Geometry check sheet. Reference: the model listing, model coordinates, mm. A direction names the side the tool comes from. Give positions to 0.01 mm unless a question says otherwise; leave off trailing zeros. Write each loop counter-clockwise with the first axis right and the second up, starting at its lowest first coordinate (ties: lowest second). Pieces come first, ordered by that corner, then holes.
(1) Tool access check on faces 4 (the flat face through (0, 2, -9.716)), 5 (the cylindrical face through (1.93, 24.81, 2.52)), 6 (the flat face through (0, 46.05, 0)), 7 (the flat face through (1.22, -8.03, 2.08)), 8 (the flat face through (4, 0, -6)). Record the directions out of +Z, -Z, +X, -X, +Y, -Y that give a thin tool (end or side, any length) a straight path to the whole face; none if there is none.
(2) Depth check by flat-ended pin: P1, Ø5.5, axis at x = -0.5, z = 0.5, coming from the -Y side; P2, Ø2, axis at y = -9, z = 0, coming from the +X side; P3, Ø2, axis at y = -8, z = 0.5, coming from the -X side; P4, Ø1, axis at x = 3.5, z = -1.5, coming from the +Y side. Enter the tip coordinate at first touch or a pass-through.
(3) Thickness scan on line 1 along Y through (x, z) = (2, -1.5); line 2 along Y through (x, z) = (2, -8); line 3 along Y through (x, z) = (2, -7). Record the ranges inside material, lowest first.
(4) Cross-section at B-B (y = 34). Record the boundary of the cut face in (x, z) (3 decimals).
(5) Mould release check, pull along Z, two halves, no side actions. Record for faces 1 (the flat face through (0, 2, 9.716)), 2 (the flat face through (-4, 4.775, 0)), 3 (the flat face through (2.413, -8, 0)): +Z half, -Z half, draft (parallel to the pull), parting line (faces both ways), or undercut.
```python
from build123d import *

# Parameters (mm, degrees)
SKETCH1_W          = 19.431
SKETCH1_H          = 19.431
EXTRUDE1_DEPTH     = 4.7752
SKETCH2_R          = 3.175
EXTRUDE2_DEPTH     = 41.275
SKETCH3_R          = 7.9375
EXTRUDE3_DEPTH     = 10.16
CHAMFER1_SIZE      = 0.635
CHAMFER2_SIZE      = 0.635
CUT_EXTRUDE1_DEPTH = 4.318
FILLET1_R          = 0.254


with BuildPart() as part:
    # Sketch1 → Extrude1 (new body)
    with BuildSketch(Plane(origin=(0, 0, 0), x_dir=(1, 0, 0), z_dir=(0, 1, 0))):
        Rectangle(SKETCH1_W, SKETCH1_H)
    extrude(amount=EXTRUDE1_DEPTH)

    # Sketch2 → Extrude2 (add)
    with BuildSketch(Plane(origin=(0, 4.7752, 0), x_dir=(-1, 0, 0), z_dir=(0, 1, 0))):
        with Locations(Location((0, 0, 0), (0, 0, 270))):  # turned: the seam where the file's is
            Circle(SKETCH2_R)
    extrude(amount=EXTRUDE2_DEPTH)

    # Sketch3 → Extrude3 (add)
    with BuildSketch(Plane.XZ):
        with Locations(Location((0, 0, 0), (0, 0, 270))):  # turned: the seam where the file's is
            Circle(SKETCH3_R)
    extrude(amount=EXTRUDE3_DEPTH)

    # Chamfer1
    chamfer1_edges = [part.edges().sort_by_distance(p)[0] for p in [
        (0, 46.0502, 3.175),
    ]]
    chamfer(chamfer1_edges, length=CHAMFER1_SIZE)

    # Sketch4 → Cut-Revolve1 (revolve, cut)
    with BuildSketch(Plane.XY, mode=Mode.PRIVATE) as cut_revolve1_sk:
        Polygon((-7.9375, 0), (-6.985, 0), (-6.985, -1.27), (-7.9375, -2.2225), align=None)
    revolve(cut_revolve1_sk.sketch.rotate(Axis((0, 0, 0), (0, -1, 0)), 270), axis=Axis((0, 0, 0), (0, -1, 0)), mode=Mode.SUBTRACT)  # turned: the seam where the file's is

    # Chamfer2
    chamfer2_edges = [part.edges().sort_by_distance(p)[0] for p in [
        (0, -10.16, 7.9375),
    ]]
    chamfer(chamfer2_edges, length=CHAMFER2_SIZE)

    # Sketch5 → Cut-Extrude1 (cut)
    with BuildSketch(Plane.XZ.offset(10.16)):
        Polygon((0, -2.786292399), (2.413, -1.3931462), (2.413, 1.3931462), (0, 2.786292399), (-2.413, 1.3931462), (-2.413, -1.3931462), align=None)
    extrude(amount=-CUT_EXTRUDE1_DEPTH, mode=Mode.SUBTRACT)

    # Fillet1
    fillet1_edges = [part.edges().sort_by_distance(p)[0] for p in [
        (9.7155, 4.7752, 0),
        (0, 4.7752, -9.7155),
        (-9.7155, 4.7752, 0),
        (0, 0, -9.7155),
        (9.7155, 0, 0),
        (0, 0, 9.7155),
        (-9.7155, 0, 0),
        (0, 4.7752, 9.7155),
        (-9.7155, 2.3876, -9.7155),
        (9.7155, 2.3876, -9.7155),
        (9.7155, 2.3876, 9.7155),
        (-9.7155, 2.3876, 9.7155),
    ]]
    fillet(fillet1_edges, radius=FILLET1_R)


solid = part.part
```
Reply:
1. face 4: -Z, +X, -X, +Y, -Y
1. face 5: +Y
1. face 6: +Z, -Z, +X, -X, +Y
1. face 7: -Y
1. face 8: none
2. P1: stops at y = -10.16
2. P2: stops at x = 7.94
2. P3: stops at x = -7.94
2. P4: stops at y = 4.78
3. line 1: y = -5.84 to 46.05
3. line 2: y = 0 to 4.78
3. line 3: y = -10.16 to -1.57, 0 to 4.78
4. outline: circle Ø6.35 at (0, 0)
5. face 1: +Z half
5. face 2: draft
5. face 3: undercut
